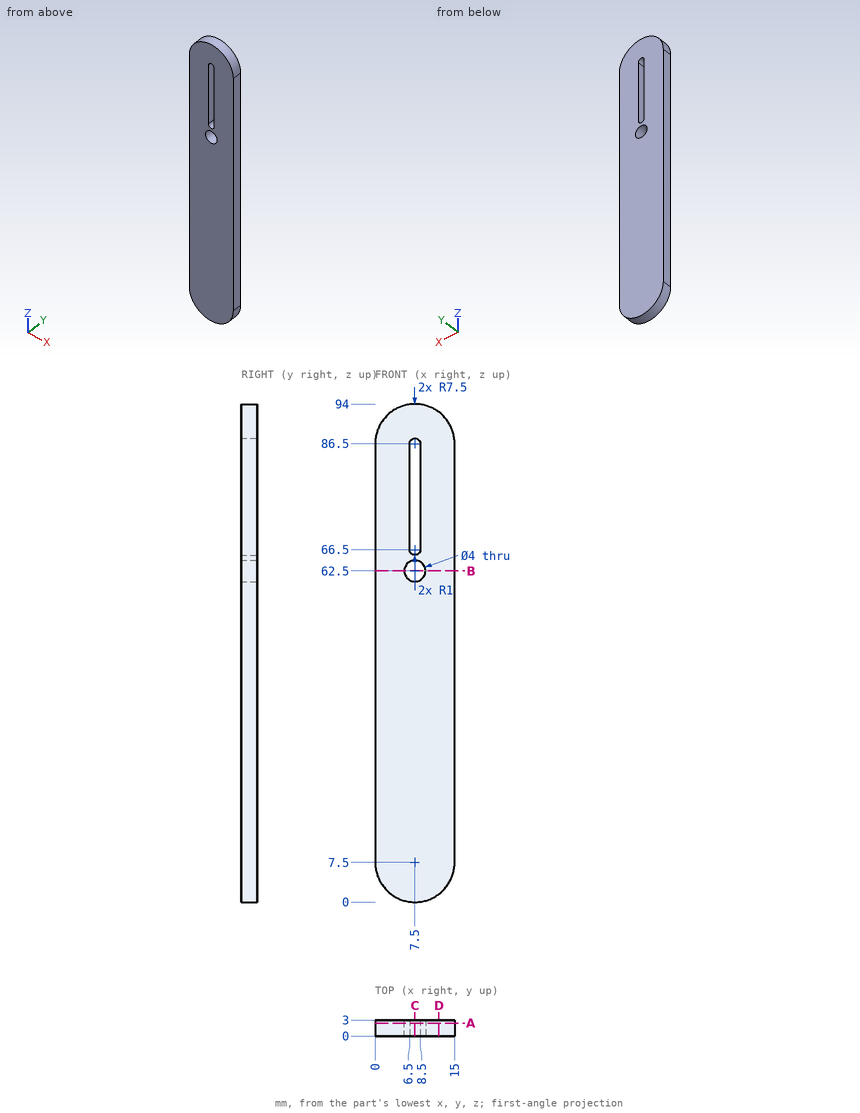
Here's the drawing with two shaded views (mm, measured from the low corner). I have some questions. Coordinates: 2 decimals unless noted, no trailing zeros. Write each loop counter-clockwise with the first axis right and the second up, starting at its lowest first coordinate (ties: lowest second). Pieces come first, ordered by that corner, then holes. Notation, with made-up numbers: (74, 67.25) -> (131, 67.25) arc R27 ccw to (131, 85.25) -> close; hole circle Ø11 at (-15.5, 81). An arc over 180 degrees is marked (long way). One line per question, with ' | ' between items. Start each with the question number.
1. If we section it at C-C (x = 7.5): Please give me the cut outline in (y, z), and give its area (3 significant figures).
2. If we section it at D-D (x = 12): Please give me the cut outline in (y, z).
3. If we section it at B-B (z = 62.5): Please give me the cut outline in (x, y), and give its area (3 significant figures).
4. If we section it at A-A (y = 2.45): Please give me the cut outline in (x, z), and give its area (3 significant figures).
5. Please list where these lines run through material, in increasing order: line 1 along Z through (x, y) = (7.5, 1.1); line 2 along X through (y, z) = (1.75, 77.5); line 3 along Z through (x, y) = (6.25, 0.3).
Return value:
1) outline: (0, 0) -> (3, 0) -> (3, 60.5) -> (0, 60.5) -> close; (0, 64.5) -> (3, 64.5) -> (3, 65.5) -> (0, 65.5) -> close; (0, 87.5) -> (3, 87.5) -> (3, 94) -> (0, 94) -> close | area: 204 mm²
2) outline: (0, 1.5) -> (3, 1.5) -> (3, 92.5) -> (0, 92.5) -> close
3) outline: (0, 0) -> (5.5, 0) -> (5.5, 3) -> (0, 3) -> close; (9.5, 0) -> (15, 0) -> (15, 3) -> (9.5, 3) -> close | area: 33.0 mm²
4) outline: (0, 7.5) arc R7.5 ccw to (15, 7.5) -> (15, 86.5) arc R7.5 ccw to (0, 86.5) -> close; hole circle Ø4 at (7.5, 62.5); hole (6.5, 66.5) arc R1 ccw to (8.5, 66.5) -> (8.5, 86.5) arc R1 ccw to (6.5, 86.5) -> close | area: 1,310 mm²
5) line 1: z = 0 to 60.5, 64.5 to 65.5, 87.5 to 94 | line 2: x = 0 to 6.5, 8.5 to 15 | line 3: z = 0.1 to 60.94, 64.06 to 93.9
